For this review, take the finished solid that the model builds, in its own axes (mm). Coordinates: 2 decimals unless noted, no trailing zeros. Loops run counter-clockwise (first coordinate to the right, second up) from the corner with the lowest first, then second, coordinate; pieces in that order, holes last. Notation, with made-up numbers: M -24.75,77.5 L -16.75,77.5 A33 ccw -16.75,112.5 Z; hole C 32.5,79 d11. An arc over 180 degrees is marked long. Write item = value, one per line.
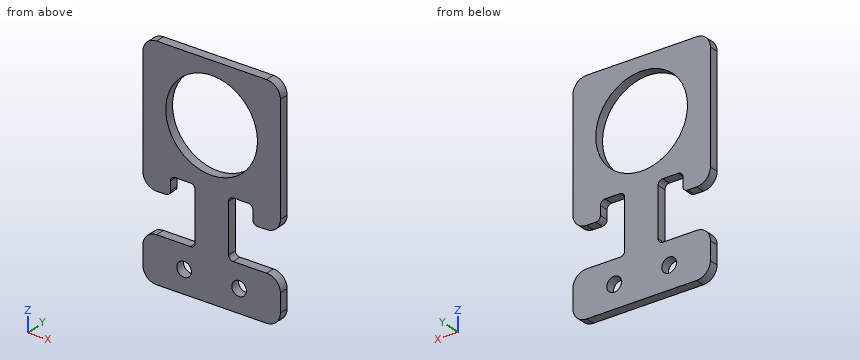
from build123d import *

# Parameters (mm, degrees)
SM_BASE_FLANGE_1_DEPTH = 2
CUT_EXTRUDE_1_DEPTH    = 10
FILLET_1_R             = 3
FILLET_2_R             = 1
CUT_EXTRUDE_3_DEPTH    = 10


# Sheet-metal steps are written as plain solids
with BuildPart() as part:
    # Sketch 1 → 基体-法兰1 (new body)
    with BuildSketch(Plane(origin=(0, 0, 0), x_dir=(1, 0, 0), z_dir=(0, 1, 0))):
        Polygon((15, 15), (9, 15), (9, 11), (3.7, 11), (3.7, 15), (3.7, 23.7), (15, 23.7), (15, 33.7), (-15, 33.7), (-15, 23.7), (-3.6, 23.7), (-3.6, 15), (-3.6, 11), (-9, 11), (-9, 15), (-15, 15), (-15, -15), (15, -15), align=None)
    extrude(amount=-SM_BASE_FLANGE_1_DEPTH)

    # 草图6 → 切除-拉伸1 (cut)
    with BuildSketch(Plane(origin=(0, 0, 0), x_dir=(1, 0, 0), z_dir=(0, 1, 0))):
        with BuildLine():
            Line((-7.6, 28.7), (-6, 28.7))
            Line((-6, 28.7), (-4.4, 28.7))
            ThreePointArc((-4.4, 28.7), (-6, 30.3), (-7.6, 28.7))
        make_face()
        with BuildLine():
            Line((-4.4, 28.7), (-6, 28.7))
            Line((-6, 28.7), (-7.6, 28.7))
            ThreePointArc((-7.6, 28.7), (-6, 27.1), (-4.4, 28.7))
        make_face()
        with BuildLine():
            ThreePointArc((7.6, 28.7), (6, 30.3), (4.4, 28.7))
            Line((4.4, 28.7), (6, 28.7))
            Line((6, 28.7), (7.6, 28.7))
        make_face()
        with BuildLine():
            Line((6, 28.7), (4.4, 28.7))
            ThreePointArc((4.4, 28.7), (6, 27.1), (7.6, 28.7))
            Line((7.6, 28.7), (6, 28.7))
        make_face()
    extrude(amount=-CUT_EXTRUDE_1_DEPTH, mode=Mode.SUBTRACT)

    # 圆角1
    fillet_1_edges = [part.edges().sort_by_distance(p)[0] for p in [
        (15, -1, 15),
        (-15, -1, 15),
        (-15, -1, -15),
        (-15, -1, -23.7),
        (-15, -1, -33.7),
        (15, -1, -33.7),
        (15, -1, -23.7),
        (15, -1, -15),
    ]]
    fillet(fillet_1_edges, radius=FILLET_1_R)

    # 圆角2
    fillet_2_edges = [part.edges().sort_by_distance(p)[0] for p in [
        (-9, -1, -15),
        (-9, -1, -11),
        (-3.6, -1, -11),
        (-3.6, -1, -23.7),
        (3.7, -1, -23.7),
        (3.7, -1, -11),
        (9, -1, -11),
        (9, -1, -15),
    ]]
    fillet(fillet_2_edges, radius=FILLET_2_R)

    # 草图7 → 切除-拉伸3 (cut)
    with BuildSketch(Plane(origin=(0, 0, 0), x_dir=(1, 0, 0), z_dir=(0, 1, 0))):
        with BuildLine():
            ThreePointArc((-10, -2), (0, -12), (10, -2))
            Line((10, -2), (-10, -2))
        make_face()
        with BuildLine():
            Line((-10, -2), (10, -2))
            ThreePointArc((10, -2), (0, 8), (-10, -2))
        make_face()
    extrude(amount=-CUT_EXTRUDE_3_DEPTH, mode=Mode.SUBTRACT)


solid = part.part
Q1. Add section C-C (x = 6). Write out the cut boundary in (y, z), and give its area (3 significant figures).
Solved:
outline = M -2,-33.7 L 0,-33.7 L 0,-30.3 L -2,-30.3 Z; M -2,-27.1 L 0,-27.1 L 0,-23.7 L -2,-23.7 Z; M -2,-11 L 0,-11 L 0,-6 L -2,-6 Z; M -2,10 L 0,10 L 0,15 L -2,15 Z
area = 33.6 mm²
Q2. Add section A-A (z = 10). Write out the cut boundary in (x, y).
Solved:
outline = M -15,-2 L -6,-2 L -6,0 L -15,0 Z; M 6,-2 L 15,-2 L 15,0 L 6,0 Z
Q3. Add section B-B (z = -28.7). Write out the cut boundary in (x, y), and give its area (3 significant figures).
Solved:
outline = M -15,-2 L -7.6,-2 L -7.6,0 L -15,0 Z; M -4.4,-2 L 4.4,-2 L 4.4,0 L -4.4,0 Z; M 7.6,-2 L 15,-2 L 15,0 L 7.6,0 Z
area = 47.2 mm²
Q4. For pin 1 Ø0.6 at (y, z) = (-1, -16) entering from +X; pin 2 Ø0.6 at (y, z) = (-0.5, -12.5) entering from +X; pin 3 Ø0.6 at (y, z) = (-1, -12.5) entering from -X, all flat-tipped, find the tip position at first contact; note any pin that passes through.
Solved:
pin_1 = 3.7
pin_2 = 14.99
pin_3 = -14.99
Q5. Add section D-D (x = 10.5). Write out the cut boundary in (y, z).
Solved:
outline = M -2,-33.7 L 0,-33.7 L 0,-23.7 L -2,-23.7 Z; M -2,-15 L 0,-15 L 0,15 L -2,15 Z
Q6. For line 1 along X through (y, z) = (-0.5, 2); line 2 along Z through (x, y) = (-8.5, -1.4); line 3 along Z through (x, y) = (0, -1.5), list the stretches that pass through material, from the lowest coordinate up.
Solved:
line_1 = -15 to -10, 10 to 15
line_2 = -33.7 to -23.7, -11.13 to -3.27, 7.27 to 15
line_3 = -33.7 to -8, 12 to 15
